Verification items for the finished model (mm, model axes). A direction names the side the tool comes from. Coordinates: 2 decimals unless noted, no trailing zeros. Loops run counter-clockwise (first coordinate to the right, second up) from the corner with the lowest first, then second, coordinate; pieces in that order, holes last. Notation, with made-up numbers: (84, -1) -> (127, -1) arc R11 ccw to (127, 7) -> close; hole circle Ø2 at (-25, -27.75). An arc over 180 degrees is marked (long way). Write item = value, one per line.
Autodesk Inventor part; units mm, degrees
sketch "Эскиз1" plane through (0, 0, 0) normal (0, 1, 0) x (-1, 0, 0)
  circle A0 centre (0, 0) radius 11
  circle A1 centre (5.5, -5.5) radius 1.5
  circle A2 centre (5.5, 5.5) radius 1.5
  circle A3 centre (-5.5, 5.5) radius 1.5
  circle A4 centre (-5.5, -5.5) radius 1.5
  line L0 (5.5, -5.5) -> (-5.5, -5.5) construction
  line L1 (-5.5, -5.5) -> (-5.5, 5.5) construction
  line L2 (-5.5, 5.5) -> (5.5, 5.5) construction
  line L3 (5.5, 5.5) -> (5.5, -5.5) construction
  line L4 (5.5, -5.5) -> (-5.5, 5.5) construction
  line L5 (-5.5, -5.5) -> (5.5, 5.5) construction
  circle A5 centre (0, 0) radius 2.5
  dimension "d0" = 22
  dimension "d1" = 3
  dimension "d2" = 11
  dimension "d5" = 5
extrude "Выдавливание1" add sketch "Эскиз1" along normal mid plane 2
sketch "Эскиз2" plane through (0, 1, 0) normal (0, 1, 0) x (1, 0, 0)
  circle A0 centre (0, 0) radius 5
  circle A1 centre (0, 0) radius 2.5
  dimension "d6" = 10
extrude "Выдавливание2" add sketch "Эскиз2" along normal blind 10
ref_plane "РабПлоскость1" through (0, 0, 0) normal (0.7071, 0, -0.7071) x (0, 1, 0)
properties part number "Фланцевая_муфта"
1) Material ranges on line 1 (Z direction, x = 0, y = 3.25); line 2 (Z direction, x = -5.5, y = 0.4); line 3 (Z direction, x = 6.5, y = 0.25), recorded low to high.
Ans:
line_1 = -5 to -2.5, 2.5 to 5
line_2 = -9.53 to -7, -4 to 4, 7 to 9.53
line_3 = -8.87 to -6.62, -4.38 to 4.38, 6.62 to 8.87
2) Sectioned sample at A-A, the plane x = 0. Record the cut outline in (y, z).
Ans:
outline = (-1, -11) -> (1, -11) -> (1, -5) -> (11, -5) -> (11, -2.5) -> (-1, -2.5) -> close; (-1, 2.5) -> (11, 2.5) -> (11, 5) -> (1, 5) -> (1, 11) -> (-1, 11) -> close
3) Depth check by flat-ended pin: pin 1 Ø1.5 at (x, z) = (-2, -8) entering from +Y; pin 2 Ø4 at (x, z) = (5.5, -5.5) entering from -Y; pin 3 Ø4 at (x, y) = (2, 8) entering from +Z. Enter the tip coordinate at first touch or a pass-through.
Ans:
pin_1 = 1
pin_2 = -1
pin_3 = 5
4) Sectioned sample at B-B, the plane z = -1.25. Record the cut outline in (x, y).
Ans:
outline = (-10.93, -1) -> (-2.17, -1) -> (-2.17, 11) -> (-4.84, 11) -> (-4.84, 1) -> (-10.93, 1) -> close; (2.17, -1) -> (10.93, -1) -> (10.93, 1) -> (4.84, 1) -> (4.84, 11) -> (2.17, 11) -> close
5) Sectioned sample at C-C, the plane x = 5.5. Record the cut outline in (y, z), plus the area to 3 significant figures.
Ans:
outline = (-1, -9.53) -> (1, -9.53) -> (1, -7) -> (-1, -7) -> close; (-1, -4) -> (1, -4) -> (1, 4) -> (-1, 4) -> close; (-1, 7) -> (1, 7) -> (1, 9.53) -> (-1, 9.53) -> close
area = 26.1 mm2
6) Sectioned sample at D-D, the plane z = 5.5. Record the cut outline in (x, y), plus the area to 3 significant figures.
Ans:
outline = (-9.53, -1) -> (-7, -1) -> (-7, 1) -> (-9.53, 1) -> close; (-4, -1) -> (4, -1) -> (4, 1) -> (-4, 1) -> close; (7, -1) -> (9.53, -1) -> (9.53, 1) -> (7, 1) -> close
area = 26.1 mm2
7) Tool access check on faces 5 (the face through (-2, 1, -5)), 6 (the face through (2, 11, 2)). Record the directions out of +Z, -Z, +X, -X, +Y, -Y that give a thin tool (end or side, any length) a straight path to the whole face; none if there is none.
Ans:
face_5 = +Y
face_6 = +Z, -Z, +X, -X, +Y
8) Release check for a two-part mould opening along X. For faces 1 (the face through (-4.3, 0, -4.6)), 2 (the face through (-4.3, 0, 4.6)), 3 (the face through (0, -1, 3)), 4 (the face through (-1.08, 5.93, -4.88)) record: pulls with the +X half, pulls with the -X half, needs draft (parallel to the pull), parting line crosses it, or undercut.
Ans:
face_1 = undercut
face_2 = undercut
face_3 = needs draft
face_4 = parting line crosses it
